Model file for the job. Use its own axes, mm. A direction names the side the tool comes from. Coordinates: 2 decimals unless noted, no trailing zeros. Write each loop counter-clockwise with the first axis right and the second up, starting at its lowest first coordinate (ties: lowest second). Pieces come first, ordered by that corner, then holes. Notation, with made-up numbers: M 38.5,29.25 L 91.5,29.25 A27 cw 91.5,64.25 Z; hole C 69,-33 d5. An arc over 180 degrees is marked long. One line per question, with ' | ' between items. Start each with the question number.
(1) Flat gauge pins, fed straight in: pin 1 Ø1 at (x, y) = (-1.5, 1) entering from -Z; pin 2 Ø1 at (x, y) = (-1.5, 5.5) entering from -Z; pin 3 Ø3 at (y, z) = (0, 4.5) entering from -X. Where does each tip first touch, or does it go through?
(2) Cut at B-B (x = 0). Write the cut outline in (y, z).
(3) Two-plate mould, pull along Y, no slides. Class faces 1 (the face through (3, 7, 0)), 2 (the face through (-6, 6, 0)), 3 (the face through (-1.42, 5, 3.92)): +Y half, -Y half, draft (parallel to the pull), parting line (faces both ways), or undercut.
(4) Tool access for faces 4 (the face through (-0.867, 2.465, 3.905)), 5 (the face through (3, -2, 0)): list every direction of +Z, -Z, +X, -X, +Y, -Y with a clear straight run to the whole face (end or side of a thin tool).
(5) Cut at C-C (y = 2). Write the cut outline in (x, z) (1 decimal).
(6) Cut at D-D (z = 3.5). Write the cut outline in (x, y).
(7) Wall check: probe 1 along Z at (x, y) = (0, 3.25); probe 2 along Y at (x, z) = (5.25, -0.75). Give the ranges that are in metal, low to high.
(8) Cut at A-A (z = 0). Write the cut outline in (x, y).
from build123d import *

# Parameters (mm, degrees)
SKETCH1_R           = 4
BOSS_EXTRUDE1_DEPTH = 5
SKETCH2_R           = 6
BOSS_EXTRUDE2_DEPTH = 2
SKETCH3_R           = 2.2225
CUT_EXTRUDE1_DEPTH  = 10


with BuildPart() as part:
    # Sketch1 → Boss-Extrude1 (new body)
    with BuildSketch(Plane(origin=(0, 0, 0), x_dir=(1, 0, 0), z_dir=(0, 1, 0))):
        Circle(SKETCH1_R)
    extrude(amount=BOSS_EXTRUDE1_DEPTH)

    # Sketch2 → Boss-Extrude2 (add)
    with BuildSketch(Plane(origin=(0, 5, 0), x_dir=(1, 0, 0), z_dir=(0, 1, 0))):
        Circle(SKETCH2_R)
    boss_extrude2 = extrude(amount=BOSS_EXTRUDE2_DEPTH)

    # Mirror1: Boss-Extrude2 across plane
    add(boss_extrude2.mirror(Plane(origin=(0, 2.5, 0), x_dir=(0, 0, 1), z_dir=(0, -1, 0))))

    # Sketch3 → Cut-Extrude1 (cut, through all)
    with BuildSketch(Plane(origin=(0, 7, 0), x_dir=(1, 0, 0), z_dir=(0, 1, 0))):
        Circle(SKETCH3_R)
    extrude(amount=-CUT_EXTRUDE1_DEPTH, mode=Mode.SUBTRACT)


solid = part.part
Filled in:
1) pin 1: z = -3.87 | pin 2: z = -5.92 | pin 3: x = -5.2
2) outline: M -2,-6 L 0,-6 L 0,-4 L 5,-4 L 5,-6 L 7,-6 L 7,-2.22 L -2,-2.22 Z; M -2,2.22 L 7,2.22 L 7,6 L 5,6 L 5,4 L 0,4 L 0,6 L -2,6 Z
3) face 1: +Y half | face 2: draft | face 3: undercut
4) face 4: none | face 5: +Z, -Z, +X, -X, -Y
5) outline: C 0,0 d8; hole C 0,0 d4.4
6) outline: M -4.87,-2 L 4.87,-2 L 4.87,0 L 1.94,0 L 1.94,5 L 4.87,5 L 4.87,7 L -4.87,7 L -4.87,5 L -1.94,5 L -1.94,0 L -4.87,0 Z
7) probe 1: -4 to -2.22, 2.22 to 4 | probe 2: -2 to 0, 5 to 7
8) outline: M -6,-2 L -2.22,-2 L -2.22,7 L -6,7 L -6,5 L -4,5 L -4,0 L -6,0 Z; M 2.22,-2 L 6,-2 L 6,0 L 4,0 L 4,5 L 6,5 L 6,7 L 2.22,7 Z
